Design review of the part built by this model. Coordinates are the model's own, in mm. A direction names the side the tool comes from. Give positions to 0.01 mm unless a question says otherwise; leave off trailing zeros. Write each loop counter-clockwise with the first axis right and the second up, starting at its lowest first coordinate (ties: lowest second). Pieces come first, ordered by that corner, then holes. Notation, with made-up numbers: M 56,-10 L 79,-10 A24 ccw 79,4 Z; hole C 31.25,-9 d9. An arc over 180 degrees is marked long. Answer in a Markdown table with one row per item.
```python
from build123d import *

# Parameters (mm, degrees)
F0_W     = 127
F0_H     = 12.7
F1_DEPTH = 88.9
F2_W     = 12.7
F2_H     = 31.75
F3_DEPTH = 88.9
F4_W     = 16.51
F4_H     = 29.21
F5_DEPTH = 5.08
F6_W     = 63.5
F6_H     = 31.75
F7_DEPTH = 19.05
F8_W     = 30.48
F8_H     = 2.54
F9_DEPTH = 5.08
F10_R    = 12.7


with BuildPart() as f1:
    # F0 (on Front) → F1 (new body)
    with BuildSketch(Plane.XZ):
        with Locations((63.5, 6.35)):
            Rectangle(F0_W, F0_H)
    extrude(amount=F1_DEPTH)

    # F2 (on face) → F3 (join)
    with BuildSketch(Plane.XZ.offset(88.9)):
        Polygon((0, 44.45), (0, 12.7), (6.35, 12.7), (12.7, 12.7), (12.7, 44.45), (6.35, 44.45), align=None)
        with Locations((25.4, 28.575)):
            Rectangle(F2_W, F2_H)
        with Locations((44.45, 28.575)):
            Rectangle(F2_W, F2_H)
        with Locations((120.65, 28.575)):
            Rectangle(F2_W, F2_H)
    extrude(amount=-F3_DEPTH)

    # F4 (on face) → F5 (join)
    with BuildSketch(Plane.XZ.offset(88.9)):
        with Locations((59.055, 27.305)):
            Rectangle(F4_W, F4_H)
        with Locations((106.045, 27.305)):
            Rectangle(F4_W, F4_H)
    extrude(amount=-F5_DEPTH)

    # F6 (on face) → F7 (join)
    with BuildSketch(Plane(origin=(0, 0, 0), x_dir=(-1, 0, 0), z_dir=(0, 1, 0))):
        with Locations((-82.55, 28.575)):
            Rectangle(F6_W, F6_H)
    extrude(amount=-F7_DEPTH)

    # F8 (on face) → F9 (join)
    with BuildSketch(Plane.XZ.offset(88.9)):
        with Locations((82.55, 13.97)):
            Rectangle(F8_W, F8_H)
    extrude(amount=-F9_DEPTH)

    # F10
    f10_edges = [f1.edges().sort_by_distance(p)[0] for p in [
        (67.31, -86.36, 41.91),
        (97.79, -86.36, 41.91),
    ]]
    fillet(f10_edges, radius=F10_R)


solid = f1.part
```
1) To check wall thickness, follow probe 1 along X at (y, z) = (-67.5, 39); probe 2 along X at (y, z) = (-10, 34.5); probe 3 along Z at (x, y) = (94.5, -24). State the ranges of each line that lie inside material, in increasing order. Write a range as [from, to].
Geometry says:
| item | result |
|---|---|
| probe 1 | [0, 12.7], [19.05, 31.75], [38.1, 50.8], [114.3, 127] |
| probe 2 | [0, 12.7], [19.05, 31.75], [38.1, 127] |
| probe 3 | [0, 12.7] |
2) The part is to be moulded in two halves that separate along X. For faces 5 (the face through (97.79, -86, 22)), 6 (the face through (0, -45, 23)), 7 (the face through (67.31, -86, 22)), 8 (the face through (6, -45, 44.45)), say which applies: released by +X, released by -X, zero draft, split by the parting line, or undercut.
Geometry says:
| item | result |
|---|---|
| face 5 | undercut |
| face 6 | released by -X |
| face 7 | undercut |
| face 8 | zero draft |
3) Insertion check: P1, Ø1.1, axis at x = 113, y = -87, coming from the +Z side; P2, Ø4, axis at x = 81, y = -86, coming from the +Z side; P3, Ø19, axis at x = 67, y = -44, coming from the +Z side. Each pin has a flat end and moves straight along its axis. Give the tip position at first contact, or say it passes through.
Geometry says:
| item | result |
|---|---|
| P1 | z = 41.91 |
| P2 | z = 15.24 |
| P3 | z = 12.7 |
4) Add section D-D (x = 82). Write out the cut boundary in (y, z), and give its area (3 significant figures).
Geometry says:
| item | result |
|---|---|
| outline | M -88.9,0 L 0,0 L 0,44.45 L -19.05,44.45 L -19.05,12.7 L -83.82,12.7 L -83.82,15.24 L -88.9,15.24 Z |
| area | 1,750 mm^2 |
5) Add section A-A (z = 18). Write out the cut boundary in (x, y), and give its area (3 significant figures).
Geometry says:
| item | result |
|---|---|
| outline | M 0,-88.9 L 12.7,-88.9 L 12.7,0 L 0,0 Z; M 19.05,-88.9 L 31.75,-88.9 L 31.75,0 L 19.05,0 Z; M 38.1,-88.9 L 67.31,-88.9 L 67.31,-83.82 L 50.8,-83.82 L 50.8,-19.05 L 114.3,-19.05 L 114.3,-83.82 L 97.79,-83.82 L 97.79,-88.9 L 127,-88.9 L 127,0 L 38.1,0 Z |
| area | 5,890 mm^2 |
6) Add section C-C (x = 66). Write out the cut boundary in (y, z).
Geometry says:
| item | result |
|---|---|
| outline | M -88.9,0 L 0,0 L 0,44.45 L -19.05,44.45 L -19.05,12.7 L -83.82,12.7 L -83.82,34.83 L -88.9,34.83 Z |
7) Add section B-B (y = -32.5). Write out the cut boundary in (x, z).
Geometry says:
| item | result |
|---|---|
| outline | M 0,0 L 127,0 L 127,44.45 L 114.3,44.45 L 114.3,12.7 L 50.8,12.7 L 50.8,44.45 L 38.1,44.45 L 38.1,12.7 L 31.75,12.7 L 31.75,44.45 L 19.05,44.45 L 19.05,12.7 L 12.7,12.7 L 12.7,44.45 L 0,44.45 Z |
8) For faces 1 (the face through (53, -86, 41.91)), 2 (the face through (83, -14, 44.45)), 3 (the face through (50.8, -54, 28)), 4 (the face through (31.75, -45, 28)), list the 3-axis set-ups (+Z, -Z, +X, -X, +Y, -Y) from which the entire face can be reached by the end or side of a thin tool; tool diameter is ignored.
Geometry says:
| item | result |
|---|---|
| face 1 | +Z, -Y |
| face 2 | +Z, +X, -X, +Y, -Y |
| face 3 | +Z |
| face 4 | +Z, +Y, -Y |
